Here's how the part is built. I have some questions about the finished solid (model axes, mm). A direction names the side the tool comes from. Coordinates: 2 decimals unless noted, no trailing zeros. Order: outer loops, then holes, each group sorted by start corner. A loop starts at its lowest first (then second) coordinate and runs counter-clockwise, first axis right, second up. Notation, with made-up numbers: (-12.5, 50.5) -> (26.5, 50.5) arc R19 ccw to (26.5, 75.5) -> close; hole circle Ø1 at (26, 23.5). An arc over 180 degrees is marked (long way). One line per item, written item: value. Start each with the question number.
```python
from build123d import *

# Parameters (mm, degrees)
SKETCH1_W                      = 35.56
SKETCH1_H                      = 50.8
BOSS_EXTRUDE1_DEPTH            = 9.525
SKETCH2_W                      = 25.4
SKETCH2_H                      = 45.72
CUT_EXTRUDE2_DEPTH             = 5.08
TAP_DRILL_FOR_M2_5X0_45_TAP1_D = 2.05
SKETCH13_W                     = 25.4
SKETCH13_H                     = 3.175
BOSS_EXTRUDE2_DEPTH            = 28.575
CUT_EXTRUDE3_DEPTH             = 73.778867812
FILLET1_R                      = 6.35
M5_CLEARANCE_HOLE1_D           = 5.3
M5_CLEARANCE_HOLE1_CSINK_D     = 5.55
M5_CLEARANCE_HOLE1_CSINK_ANGLE = 90
RIB7_REACH                     = 67.774
SKETCH14_WALL_W                = 162.819779212
SKETCH14_WALL_H                = 2.54
RIB8_START                     = -2.54
RIB8_DEPTH                     = 2.54
RIB9_REACH                     = 67.774
SKETCH17_WALL_W                = 162.819779212
SKETCH17_WALL_H                = 2.54
RIB10_START                    = -2.54
RIB10_DEPTH                    = 2.54
FILLET2_R                      = 3.175
FILLET3_R                      = 3.175


# Read off the part's stored shape, not the designer's step: Rib8, Rib10
with BuildPart() as part:
    # Sketch1 → Boss-Extrude1 (new body)
    with BuildSketch(Plane.XY):
        with Locations((-17.78, 25.4)):
            Rectangle(SKETCH1_W, SKETCH1_H)
    extrude(amount=BOSS_EXTRUDE1_DEPTH)

    # Sketch2 → Cut-Extrude2 (cut)
    with BuildSketch(Plane.XY.offset(9.525)):
        with Locations((-17.78, 27.94)):
            Rectangle(SKETCH2_W, SKETCH2_H)
    extrude(amount=-CUT_EXTRUDE2_DEPTH, mode=Mode.SUBTRACT)

    # Tap Drill for M2.5x0.45 Tap1 (through all)
    with Locations(Plane(origin=(0, 0, 0), x_dir=(-1, 0, 0), z_dir=(0, 0, -1))):
        with Locations((2.792369004, 43.087106138), (2.792369004, 26.092979092), (2.792369004, 9.105182099), (9.290740849, 2.822744672), (26.292369004, 2.787106138), (32.780032006, 9.105182099), (32.792369004, 26.087106138), (32.792369004, 43.087106138)):
            Hole(TAP_DRILL_FOR_M2_5X0_45_TAP1_D / 2)

    # Sketch13 → Boss-Extrude2 (add)
    with BuildSketch(Plane(origin=(0, 0, 0), x_dir=(-1, 0, 0), z_dir=(0, 0, -1))):
        with Locations((17.78, 37.677545037)):
            Rectangle(SKETCH13_W, SKETCH13_H)
        with Locations((17.78, 14.502545037)):
            Rectangle(SKETCH13_W, SKETCH13_H)
    extrude(amount=BOSS_EXTRUDE2_DEPTH)

    # Sketch8 → Cut-Extrude3 (cut, through all)
    with BuildSketch(Plane.XY.offset(9.525)):
        Polygon((-5.178964387, 50.8), (0, 44.591495864), (0, 50.8), align=None)
        Polygon((-35.56, 44.706622517), (-35.56, 50.8), (-30.402645731, 50.8), align=None)
        Polygon((-35.56, 5.970049098), (-35.56, 0), (-30.492594088, 0), align=None)
        Polygon((-5.092594088, -0.031324356), (0, 0), (0, 5.970049098), align=None)
    extrude(amount=-CUT_EXTRUDE3_DEPTH, mode=Mode.SUBTRACT)

    # Fillet1
    fillet1_edges = [part.edges().sort_by_distance(p)[0] for p in [
        (-30.48, 5.08, 6.985),
        (-5.08, 5.08, 6.985),
    ]]
    fillet(fillet1_edges, radius=FILLET1_R)

    # M5 Clearance Hole1 (through all)
    with Locations(Plane(origin=(-17.78, 39.265045037, -7.14375), x_dir=(0, 0, 1), z_dir=(0, 1, 0))):
        with Locations((0, 0), (-14.2875, 0)):
            CounterSinkHole(M5_CLEARANCE_HOLE1_D / 2, M5_CLEARANCE_HOLE1_CSINK_D / 2, counter_sink_angle=M5_CLEARANCE_HOLE1_CSINK_ANGLE)

    # Sketch14 wall → Rib7 (add, up to next)
    with BuildSketch(Plane(origin=(-30.48, 9.740045037, -14.2875), x_dir=(0, -0.216930457819, 0.976187060184), z_dir=(0, 0.976187060184, 0.216930457819)), mode=Mode.PRIVATE) as rib7_sk1:
        with Locations((0, 1.27)):
            Rectangle(SKETCH14_WALL_W, SKETCH14_WALL_H)
    rib7_tool1 = extrude(rib7_sk1.sketch, amount=RIB7_REACH, mode=Mode.PRIVATE) - part.part
    add(rib7_tool1.solids().sort_by_distance((-30.48, 9.740045037, -14.2875))[0])

    # Rib8 outline → Rib8 (add)
    with BuildSketch(Plane(origin=(-5.08, 0, 0), x_dir=(0, 0, -1), z_dir=(1, 0, 0)).offset(RIB8_START)):
        Polygon((0, 6.565045037), (28.575, 12.915045037), (0, 12.915045037), align=None)
    extrude(amount=RIB8_DEPTH)

    # Sketch17 wall → Rib9 (add, up to next)
    with BuildSketch(Plane(origin=(-5.08, 42.440045037, -14.2875), x_dir=(0, 0.216930457819, 0.976187060184), z_dir=(0, -0.976187060184, 0.216930457819)), mode=Mode.PRIVATE) as rib9_sk1:
        with Locations((0, 1.27)):
            Rectangle(SKETCH17_WALL_W, SKETCH17_WALL_H)
    rib9_tool1 = extrude(rib9_sk1.sketch, amount=RIB9_REACH, mode=Mode.PRIVATE) - part.part
    add(rib9_tool1.solids().sort_by_distance((-5.08, 42.440045037, -14.2875))[0])

    # Rib10 outline → Rib10 (add)
    with BuildSketch(Plane.ZY.offset(30.48).offset(RIB10_START)):
        Polygon((0, 45.615045037), (-28.575, 39.265045037), (0, 39.265045037), align=None)
    extrude(amount=RIB10_DEPTH)

    # Fillet2
    fillet2_edges = [part.edges().sort_by_distance(p)[0] for p in [
        (-27.94, 12.915045037, -14.2875),
        (-7.62, 12.915045037, -14.2875),
    ]]
    fillet(fillet2_edges, radius=FILLET2_R)

    # Fillet3
    fillet3_edges = [part.edges().sort_by_distance(p)[0] for p in [
        (-7.62, 39.265045037, -14.2875),
        (-27.94, 39.265045037, -14.2875),
    ]]
    fillet(fillet3_edges, radius=FILLET3_R)


solid = part.part
```
Q1. Imagine slicing it at C-C (y = 38.5). Write out the boundary of the cut face in (x, z) (3 decimals), plus the area to 3 significant figures.
Q2. For P1, Ø1, axis at x = -11, y = 22, coming from the +Z side (3 decimals); P2, Ø7.5, axis at y = 13, z = -11.5, coming from the -X side; P3, Ø4, axis at x = -15, z = -14, coming from the +Y side; P4, Ø3, axis at x = -17.78, z = -7.14, coming from the +Y side, each with a flat end and sliding along its axis, tell me the tip position at first contact or that it passes through.
Q3. Imagine slicing it at B-B (z = -15). Write out the boundary of the cut face in (x, y) (3 decimals).
Q4. I need wall thicknesses on line 1 (X direction, y = 43, z = 4); line 2 (Y direction, x = -21, z = -0.5); line 3 (X direction, y = 43.5, z = 3). Which ranges of each line are inside material? Lowest first, please.
Q5. Imagine slicing it at D-D (y = 21.5). Write out the boundary of the cut face in (x, z) (3 decimals).
Q6. Imagine slicing it at A-A (x = -17.78). Count the separate pieces of the cut face and the enclosed holes in it, plus the area to 3 significant figures.
Q7. For faces 1 (the face through (-27.94, 43, -4)), 2 (the face through (-5.08, 40, -11)), 3 (the face through (-30.48, 13, -11)), 4 (the face through (-8.575, 12.01, -10.912)), which set-ups out of +Z, -Z, +X, -X, +Y, -Y let a thin tool reach every point of the face, with its end or its side?
Q8. If we mould it in two halves opening along Y, with no side actions, what happens to faces 5 (the face through (-18, 36.09, -14)), 6 (the face through (-2.626, 47.739, 4.829)), 7 (the face through (-15.989, 37.594, -19.478))? For each: +Y half, -Y half, draft (parallel to the pull), parting line (faces both ways), or undercut.
Completed:
1. outline: (-35.56, 0) -> (-30.48, 0) -> (-30.48, -28.575) -> (-5.08, -28.575) -> (-5.08, 0) -> (0, 0) -> (0, 9.525) -> (-5.08, 9.525) -> (-5.08, 4.445) -> (-30.48, 4.445) -> (-30.48, 9.525) -> (-35.56, 9.525) -> close; hole circle Ø5.3 at (-17.78, -21.431); hole circle Ø5.3 at (-17.78, -7.144)
1. area: 891 mm2
2. P1: stops at z = 4.445
2. P2: stops at x = -30.48
2. P3: stops at y = 39.27
2. P4: passes through
3. outline: (-30.48, 9.898) -> (-27.936, 9.898) arc R3.175 cw to (-24.765, 12.915) -> (-10.795, 12.915) arc R3.175 cw to (-7.624, 9.898) -> (-5.08, 9.898) -> (-5.08, 16.09) -> (-30.48, 16.09) -> close; (-30.48, 36.09) -> (-5.08, 36.09) -> (-5.08, 42.282) -> (-7.624, 42.282) arc R3.175 cw to (-10.795, 39.265) -> (-24.765, 39.265) arc R3.175 cw to (-27.936, 42.282) -> (-30.48, 42.282) -> close
4. line 1: x = -35.56 to -33.81, -31.77 to -3.81, -1.77 to 0
4. line 2: y = 12.92 to 16.09, 36.09 to 39.27
4. line 3: x = -35.56 to -33.73, -31.85 to -3.73, -1.85 to 0
5. outline: (-35.56, 0) -> (0, 0) -> (0, 9.525) -> (-5.08, 9.525) -> (-5.08, 4.445) -> (-30.48, 4.445) -> (-30.48, 9.525) -> (-35.56, 9.525) -> close
6. separate pieces: 5
6. enclosed holes: 0
6. area: 366 mm2
7. face 1: -Z, +Y
7. face 2: -Z, +X, +Y, -Y
7. face 3: -Z, -X, +Y, -Y
7. face 4: -Z, -Y
8. face 5: undercut
8. face 6: +Y half
8. face 7: draft
